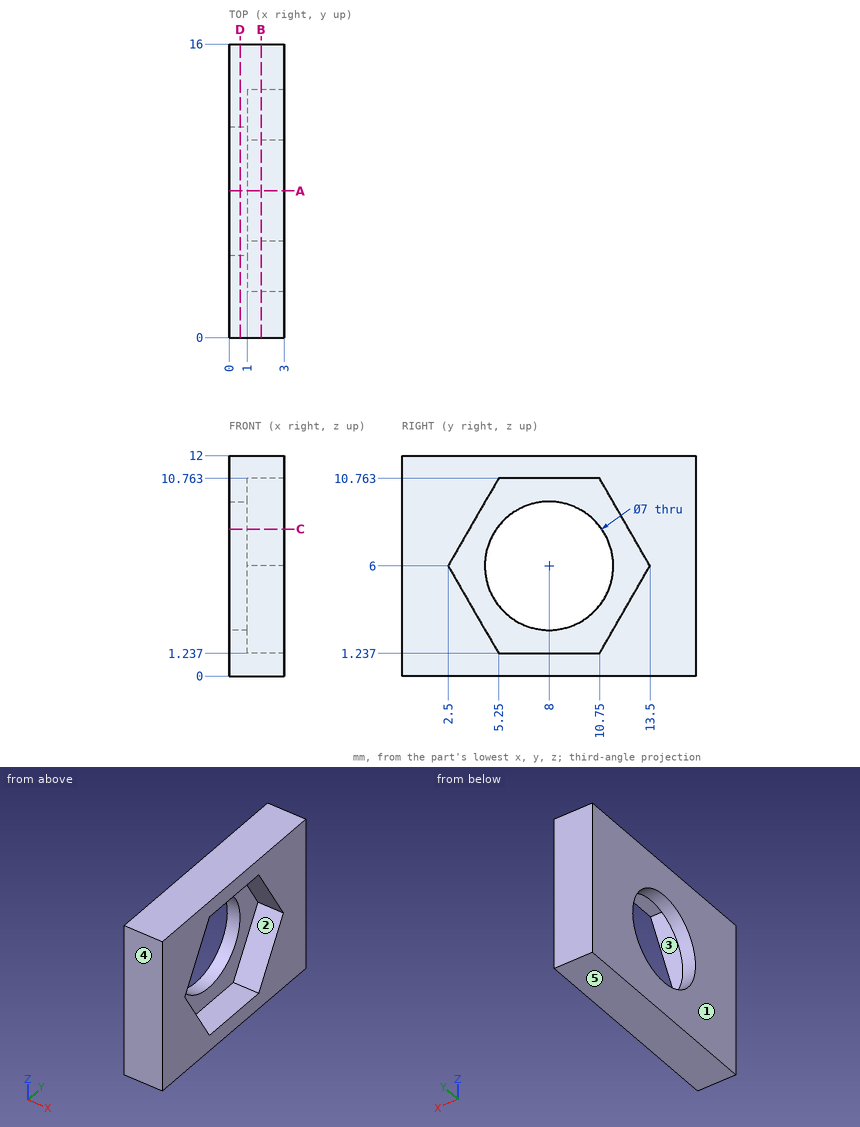
For this review, use the dimensioned drawing (mm, ordinates from the lowest corner) and the shaded views. A direction names the side the tool comes from. Round coordinates to 2 decimals unless told otherwise and drop trailing zeros. Order: outer loops, then holes, each group sorted by start corner. A loop starts at its lowest first (then second) coordinate and runs counter-clockwise, first axis right, second up.
1) Draft analysis for pull direction Y (two halves, no side actions). For the marked faces 3, 4 and 5, state which applies: released by +Y, released by -Y, zero draft, split by the parting line, or undercut.
The answers:
face 3: undercut
face 4: released by -Y
face 5: zero draft
2) Consider section D-D (x = 0.6). State the section outline as (y, z) points, plus the area to 4 significant figures.
The answers:
outline: (0, 0) - (16, 0) - (16, 12) - (0, 12) - close; hole circle Ø7 at (8, 6)
area: 153.5 mm2
3) Machinability: for the marked faces 1 and 2, which of the approach directions +Z, -Z, +X, -X, +Y, -Y give a long, thin tool a straight path to every point of the face, cutting with its end or side? Answer none if there is none.
The answers:
face 1: +Z, -Z, -X, +Y, -Y
face 2: +X
4) Consider section A-A (y = 8). State the section outline as (x, z) points.
The answers:
outline: (0, 0) - (3, 0) - (3, 1.24) - (1, 1.24) - (1, 2.5) - (0, 2.5) - close; (0, 9.5) - (1, 9.5) - (1, 10.76) - (3, 10.76) - (3, 12) - (0, 12) - close
5) Consider section C-C (z = 8). State the section outline as (x, y) points.
The answers:
outline: (0, 0) - (3, 0) - (3, 3.65) - (1, 3.65) - (1, 5.13) - (0, 5.13) - close; (0, 10.87) - (1, 10.87) - (1, 12.35) - (3, 12.35) - (3, 16) - (0, 16) - close
6) Consider section B-B (x = 1.75). State the section outline as (y, z) points.
The answers:
outline: (0, 0) - (16, 0) - (16, 12) - (0, 12) - close; hole (2.5, 6) - (5.25, 1.24) - (10.75, 1.24) - (13.5, 6) - (10.75, 10.76) - (5.25, 10.76) - close
7) Clearance check with flat-ended pins moving along their axes: pin 1 Ø6 at (y, z) = (9, 3.5) entering from -X; pin 2 Ø6.5 at (y, z) = (8, 6) entering from +X; pin 3 Ø3 at (y, z) = (6.5, 7.5) entering from +X. State where each tip first meets the part, or that it passes through.
The answers:
pin 1: stops at x = 0
pin 2: passes through
pin 3: stops at x = 1
8) For L1, parallel to Y at x = 0.6, z = 6; L2, parallel to Z at x = 2.4, y = 8; L3, parallel to X at y = 11.25, z = 4.5, list the stretches that pass through material, from the lowest coordinate up.
The answers:
L1: y = 0 to 4.5, 11.5 to 16
L2: z = 0 to 1.24, 10.76 to 12
L3: x = 0 to 1
